Here's how the part is built. I have some questions about the finished solid (model axes, mm). Face numbers are marked on the shaded views. A direction names the side the tool comes from. Give positions to 0.01 mm unless a question says otherwise; leave off trailing zeros. Write each loop counter-clockwise with the first axis right and the second up, starting at its lowest first coordinate (ties: lowest second). Pieces come first, ordered by that corner, then holes. Notation, with made-up numbers: (22.5, 14.25) -> (48.5, 14.25) arc R24 ccw to (48.5, 51.25) -> close; hole circle Ø4 at (85, 6). An arc over 180 degrees is marked (long way). Use CSV: the item, a comma, the result in double quotes. Start each with the question number.
(1) Which directions (+Z, -Z, +X, -X, +Y, -Y) give clear straight access to the entire face, cutting with the end or side of a thin tool? Please do the marked faces 1, 2, 3 and 4.
(2) Suppose I cut it at C-C on y = 4.25. List the corners of the cut face in (x, z) for me.
(3) I need wall thicknesses on L1, parallel to X at y = -2.25, z = -9.5; L2, parallel to X at y = -4.5, z = 0; L3, parallel to Z at x = -10.5, y = -4.25. Which ranges of each line are inside material? Lowest first, please. Write a range as [from, to].
(4) For pin 1 Ø1.7 at (x, y) = (-10.5, 4) entering from -Z; pin 2 Ø3 at (y, z) = (-5, 10) entering from +X, each with a flat end and sliding along its axis, tell me the tip position at first contact or that it passes through.
(5) Suppose I cut it at D-D on x = -9. List the corners of the cut face in (y, z) for me.
(6) Suppose I cut it at A-A on y = -8. Give the number of separate pieces and of enclosed holes in the cut face, plus the area to 3 significant figures.
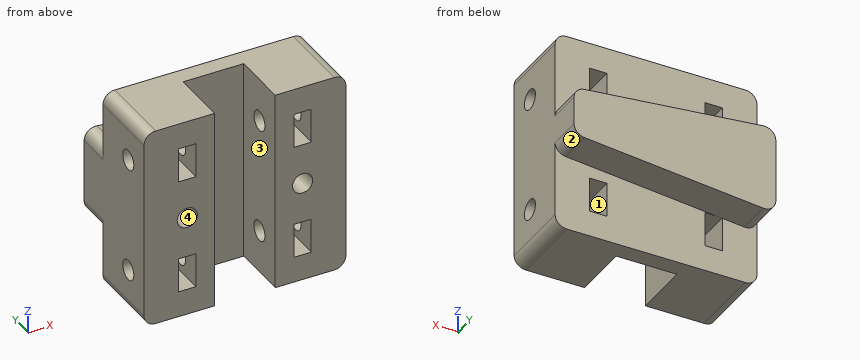
from build123d import *

# Parameters (mm, degrees)
SKETCH_1_W          = 35
SKETCH_1_H          = 35
EXTRUDE_6_DEPTH     = 3
EXTRUDE_7_DEPTH     = 6
SKETCH_6_W          = 12.25
SKETCH_6_H          = 35
EXTRUDE_8_DEPTH     = 10
FILLET_2_R          = 2
SKETCH_7_R          = 1.75
CUT_EXTRUDE_3_DEPTH = 41.388736054
SKETCH_8_W          = 3
SKETCH_8_H          = 6
CUT_EXTRUDE_4_DEPTH = 13
CUT_EXTRUDE_5_DEPTH = 4
SKETCH_12_R         = 1.75
CUT_EXTRUDE_6_DEPTH = 28.726341266


with BuildPart() as part:
    # Эскиз1 → Бобышка-Вытянуть6 (new body)
    with BuildSketch(Plane(origin=(0, 0, 0), x_dir=(1, 0, 0), z_dir=(0, 1, 0))):
        Rectangle(SKETCH_1_W, SKETCH_1_H)
    extrude(amount=EXTRUDE_6_DEPTH)

    # Эскиз5 → Бобышка-Вытянуть7 (add)
    with BuildSketch(Plane(origin=(0, 3, 0), x_dir=(1, 0, 0), z_dir=(0, 1, 0))):
        Polygon((-17.5, 7.700997512), (-17.5, 7.5), (-17.5, -7.5), (-17.5, -7.700997512), (17.5, -4.200997512), (17.5, -4), (17.5, 4), (17.5, 4.200997512), align=None)
    extrude(amount=EXTRUDE_7_DEPTH)

    # Эскиз6 → Бобышка-Вытянуть8 (add)
    with BuildSketch(Plane.XZ):
        with Locations((-11.375, 0)):
            Rectangle(SKETCH_6_W, SKETCH_6_H)
        with Locations((11.375, 0)):
            Rectangle(SKETCH_6_W, SKETCH_6_H)
    extrude(amount=EXTRUDE_8_DEPTH)

    # Скругление2
    fillet_2_edges = [part.edges().sort_by_distance(p)[0] for p in [
        (17.5, 6, 4.200997512),
        (17.5, 6, -4.200997512),
        (-17.5, 6, -7.700997512),
        (-17.5, 6, 7.700997512),
        (-17.5, -3.5, 17.5),
        (17.5, -3.5, 17.5),
        (17.5, -3.5, -17.5),
        (-17.5, -3.5, -17.5),
    ]]
    fillet(fillet_2_edges, radius=FILLET_2_R)

    # Эскиз7 → Вырез-Вытянуть3 (cut, through all)
    with BuildSketch(Plane.ZY.offset(17.5)):
        with Locations((-10, -5)):
            Circle(SKETCH_7_R)
        with Locations((10, -5)):
            Circle(SKETCH_7_R)
    extrude(amount=-CUT_EXTRUDE_3_DEPTH, mode=Mode.SUBTRACT)

    # Эскиз8 → Вырез-Вытянуть4 (cut)
    with BuildSketch(Plane.XZ.offset(10)):
        with Locations((-10, -10)):
            Rectangle(SKETCH_8_W, SKETCH_8_H)
        with Locations((10, -10)):
            Rectangle(SKETCH_8_W, SKETCH_8_H)
        with Locations((-10, 10)):
            Rectangle(SKETCH_8_W, SKETCH_8_H)
        with Locations((10, 10)):
            Rectangle(SKETCH_8_W, SKETCH_8_H)
    extrude(amount=-CUT_EXTRUDE_4_DEPTH, mode=Mode.SUBTRACT)

    # Эскиз11 → Вырез-Вытянуть5 (cut)
    with BuildSketch(Plane(origin=(0, 6.5, 0), x_dir=(1, 0, 0), z_dir=(0, 1, 0))):
        Polygon((-8.267949192, -3), (-6.535898385, 0), (-8.267949192, 3), (-11.732050808, 3), (-13.464101615, 0), (-11.732050808, -3), align=None)
        Polygon((6.535898385, 0), (8.267949192, -3), (11.732050808, -3), (13.464101615, 0), (11.732050808, 3), (8.267949192, 3), align=None)
    extrude(amount=-CUT_EXTRUDE_5_DEPTH, mode=Mode.SUBTRACT)

    # Эскиз12 → Вырез-Вытянуть6 (cut, through all)
    with BuildSketch(Plane(origin=(0, 2.5, 0), x_dir=(1, 0, 0), z_dir=(0, 1, 0))):
        with Locations(Location((-10, 0, 0), (0, 0, 270))):
            Circle(SKETCH_12_R)
        with Locations(Location((10, 0, 0), (0, 0, 270))):
            Circle(SKETCH_12_R)
    extrude(amount=-CUT_EXTRUDE_6_DEPTH, mode=Mode.SUBTRACT)


solid = part.part
Geometry says:
1,face 1,"+Y, -Y"
1,face 2,"-Z, +X, +Y"
1,face 3,"+Z, -Z, -Y"
1,face 4,"-Y"
2,outline,"(-17.5, -5.49) arc R2 ccw to (-15.3, -7.48) -> (15.7, -4.38) arc R2 ccw to (17.5, -2.39) -> (17.5, 2.39) arc R2 ccw to (15.7, 4.38) -> (-15.3, 7.48) arc R2 ccw to (-17.5, 5.49) -> close; hole (-13.46, 0) -> (-11.73, -3) -> (-8.27, -3) -> (-6.54, 0) -> (-8.27, 3) -> (-11.73, 3) -> close; hole (6.54, 0) -> (8.27, -3) -> (11.73, -3) -> (13.46, 0) -> (11.73, 3) -> (8.27, 3) -> close"
3,L1,"[-17.5, -11.5], [-8.5, -5.25], [5.25, 8.5], [11.5, 17.5]"
3,L2,"[-17.5, -11.75], [-8.25, -5.25], [5.25, 8.25], [11.75, 17.5]"
3,L3,"[-17.5, -13], [-7, -1.68], [1.68, 7], [13, 17.5]"
4,pin 1,"z = -7.09"
4,pin 2,"through"
5,outline,"(-10, -17.5) -> (3, -17.5) -> (3, -13) -> (-10, -13) -> close; (-10, -7) -> (3, -7) -> (3, -6.85) -> (9, -6.85) -> (9, 6.85) -> (3, 6.85) -> (3, 7) -> (-10, 7) -> (-10, 1.44) -> (2.5, 1.44) -> (2.5, 3) -> (6.5, 3) -> (6.5, -3) -> (2.5, -3) -> (2.5, -1.44) -> (-10, -1.44) -> close; (-10, 13) -> (3, 13) -> (3, 17.5) -> (-10, 17.5) -> close"
6,separate pieces,"2"
6,enclosed holes,"6"
6,area,"763 mm²"
